Input: part model. Units: mm. Frame: model coordinates. Face numbers are marked on the shaded views. A direction names the side the tool comes from. Give positions to 0.01 mm unless a question says otherwise; leave off trailing zeros. Loops run counter-clockwise (first coordinate to the right, second up) from the corner with the lowest first, then second, coordinate; pieces in that order, holes last. Notation, with made-up numbers: M 37.25,42.25 L 61.25,42.25 A15 cw 61.25,49.25 Z; hole C 18.25,17 d1. An arc over 180 degrees is marked long. One line per item, written item: value. Start each with the question number.
(1) Section B-B on z = 35.5. Output: boundary loops of the cut face in (x, y) (3 decimals), plus the area to 3 significant figures.
(2) Section A-A on y = 25.5. Output: boundary loops of the cut face in (x, z), plus the area to 3 significant figures.
(3) Pull-direction query (Y, two-part tool) for the marked faces 1, 2 and 3; classes: released by +Y, released by -Y, zero draft, split by the parting line, or undercut.
(4) Access query for the marked faces 4, 5 and 6. Directions: +Z, -Z, +X, -X, +Y, -Y. A direction counts if a zero-diameter tool reaches every point of the face in a straight line with its end or side. Return the directions, or none.
(5) Section C-C on x = 16. Output: boundary loops of the cut face in (y, z), plus the area to 3 significant figures.
(6) Pin query (flat end, axial travel): P1, Ø3, axis at y = 7, z = 53.5, coming from the -X side; P2, Ø7.5, axis at x = -30.988, y = 69.088, coming from the +Z side; P3, Ø5.5, axis at x = -30.99, y = -69.09, coming from the -Z side; P4, Ø1.4, axis at x = -6, z = -46.5, coming from the -Y side. Return the tip coordinate at first contact, or that it passes through.
(7) Ray query, line 1 along Y through (x, z) = (0, 145); line 2 along Y through (x, z) = (0, -23); line 3 along Z through (x, y) = (31, -51). Return the intervals inside material, ascending. Write a range as from..to.
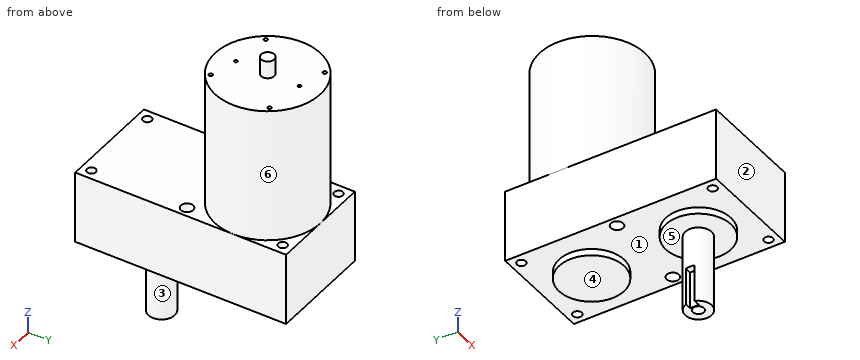
```python
from build123d import *

# Parameters (mm, degrees)
SKETCH1_W                 = 76.2
SKETCH1_H                 = 152.4
SKETCH1_R                 = 4.445
SKETCH1_R_2               = 3.175
SKETCH1_R_3               = 23.495
SKETCH1_R_4               = 9.525
SKETCH1_R_5               = 3.96875
BOSS_EXTRUDE1_DEPTH       = 52.324
SKETCH1_3_R               = 23.495
SKETCH1_3_R_2             = 9.525
BOSS_EXTRUDE2_DEPTH       = 4.826
SKETCH1_5_R               = 9.525
SKETCH1_5_R_2             = 3.96875
BOSS_EXTRUDE3_DEPTH       = 60.198
CUT_EXTRUDE1_START        = -26.924
CUT_EXTRUDE1_DEPTH        = 26.924
SKETCH4_R                 = 38.1
BOSS_EXTRUDE4_DEPTH       = 97.536
SKETCH5_R                 = 4.7625
BOSS_EXTRUDE5_DEPTH       = 12.7
F_4_40_TAPPED_HOLE1_D     = 2.2606
F_4_40_TAPPED_HOLE1_DEPTH = 7.6
F_4_40_TAPPED_HOLE1_TIP   = 0.679152758
F_6_32_TAPPED_HOLE1_D     = 2.7051
F_6_32_TAPPED_HOLE1_DEPTH = 9.39
F_6_32_TAPPED_HOLE1_TIP   = 0.81269403


with BuildPart() as part:
    # Sketch1 → Boss-Extrude1 (new body)
    # profile 1 of 5: a face of its own
    with BuildSketch(Plane.XY):
        Rectangle(SKETCH1_W, SKETCH1_H)
        with Locations((30.988, 0)):
            Circle(SKETCH1_R, mode=Mode.SUBTRACT)
        with Locations((-30.988, 69.088)):
            Circle(SKETCH1_R_2, mode=Mode.SUBTRACT)
        with Locations((-30.994242086, -69.088)):
            Circle(SKETCH1_R_2, mode=Mode.SUBTRACT)
        with Locations((0, 38.608)):
            Circle(SKETCH1_R_3, mode=Mode.SUBTRACT)
        with Locations((0, -38.608)):
            Circle(SKETCH1_R_3, mode=Mode.SUBTRACT)
        with Locations((-30.988, 0)):
            Circle(SKETCH1_R, mode=Mode.SUBTRACT)
        with Locations((30.994242086, -69.088)):
            Circle(SKETCH1_R_2, mode=Mode.SUBTRACT)
        with Locations((30.988, 69.088)):
            Circle(SKETCH1_R_2, mode=Mode.SUBTRACT)
    # profile 2 of 5: a face of its own
    with BuildSketch(Plane.XY):
        with Locations((0, 38.608)):
            Circle(SKETCH1_R_3)
    # profile 3 of 5: a face of its own
    with BuildSketch(Plane.XY):
        with Locations((0, -38.608)):
            Circle(SKETCH1_R_3)
        with Locations((0, -38.608)):
            Circle(SKETCH1_R_4, mode=Mode.SUBTRACT)
    # profile 4 of 5: a face of its own
    with BuildSketch(Plane.XY):
        with Locations((0, -38.608)):
            Circle(SKETCH1_R_4)
        with Locations((0, -38.608)):
            Circle(SKETCH1_R_5, mode=Mode.SUBTRACT)
    # profile 5 of 5: a face of its own
    with BuildSketch(Plane.XY):
        with Locations((0, -38.608)):
            Circle(SKETCH1_R_5)
    extrude(amount=BOSS_EXTRUDE1_DEPTH)

    # Sketch1_3 → Boss-Extrude2 (add)
    # profile 1 of 2: a face of its own
    with BuildSketch(Plane.XY):
        with Locations((0, 38.608)):
            Circle(SKETCH1_3_R)
    # profile 2 of 2: a face of its own
    with BuildSketch(Plane.XY):
        with Locations((0, -38.608)):
            Circle(SKETCH1_3_R)
        with Locations((0, -38.608)):
            Circle(SKETCH1_3_R_2, mode=Mode.SUBTRACT)
    extrude(amount=-BOSS_EXTRUDE2_DEPTH)

    # Sketch1_5 → Boss-Extrude3 (add)
    with BuildSketch(Plane.XY):
        with Locations((0, -38.608)):
            Circle(SKETCH1_5_R)
        with Locations((0, -38.608)):
            Circle(SKETCH1_5_R_2, mode=Mode.SUBTRACT)
    extrude(amount=-BOSS_EXTRUDE3_DEPTH)

    # Sketch2 → Cut-Extrude1 (cut)
    with BuildSketch(Plane(origin=(0, 0, -60.198), x_dir=(-1, 0, 0), z_dir=(0, 0, -1)).offset(CUT_EXTRUDE1_START)):
        with BuildLine():
            Line((8.980256121, -35.433), (4.427938354, -35.433))
            Line((4.427938354, -35.433), (4.427938354, -41.783))
            Line((4.427938354, -41.783), (8.980256121, -41.783))
            ThreePointArc((8.980256121, -41.783), (9.525, -38.608), (8.980256121, -35.433))
        make_face()
    extrude(amount=CUT_EXTRUDE1_DEPTH, mode=Mode.SUBTRACT)

    # Sketch4 → Boss-Extrude4 (add)
    with BuildSketch(Plane.XY.offset(52.324)):
        with Locations((0, 38.1)):
            Circle(SKETCH4_R)
    extrude(amount=BOSS_EXTRUDE4_DEPTH)

    # Sketch5 → Boss-Extrude5 (add)
    with BuildSketch(Plane.XY.offset(149.86)):
        with Locations((0, 38.1)):
            Circle(SKETCH5_R)
    extrude(amount=BOSS_EXTRUDE5_DEPTH)

    # 4-40 Tapped Hole1
    with Locations(Plane.XY.offset(149.86)):
        with Locations((0, 61.1), (0, 15.1)):
            Hole(F_4_40_TAPPED_HOLE1_D / 2, depth=F_4_40_TAPPED_HOLE1_DEPTH)
            with Locations((0, 0, -(F_4_40_TAPPED_HOLE1_DEPTH + F_4_40_TAPPED_HOLE1_TIP / 2))):  # 118° drill point
                Cone(0, F_4_40_TAPPED_HOLE1_D / 2, F_4_40_TAPPED_HOLE1_TIP, mode=Mode.SUBTRACT)

    # 6-32 Tapped Hole1
    with Locations(Plane.XY.offset(149.86)):
        with Locations((28.296788218, 57.913624417), (19.813624417, 9.803211782), (-28.296788218, 18.286375583), (-19.813624417, 66.396788218)):
            Hole(F_6_32_TAPPED_HOLE1_D / 2, depth=F_6_32_TAPPED_HOLE1_DEPTH)
            with Locations((0, 0, -(F_6_32_TAPPED_HOLE1_DEPTH + F_6_32_TAPPED_HOLE1_TIP / 2))):  # 118° drill point
                Cone(0, F_6_32_TAPPED_HOLE1_D / 2, F_6_32_TAPPED_HOLE1_TIP, mode=Mode.SUBTRACT)


solid = part.part
```
Output values:
1. outline: M -38.1,-76.2 L 38.1,-76.2 L 38.1,76.2 L -38.1,76.2 Z; hole C -30.988,0 d8.89; hole C -30.994,-69.088 d6.35; hole C -30.988,69.088 d6.35; hole C 30.988,0 d8.89; hole C 30.988,69.088 d6.35; hole C 30.994,-69.088 d6.35
1. area: 11,400 mm²
2. outline: M -38.1,0 L -19.5,0 L -19.5,-4.83 L 19.5,-4.83 L 19.5,0 L 38.1,0 L 38.1,52.32 L 35.96,52.32 L 35.96,149.86 L -35.96,149.86 L -35.96,52.32 L -38.1,52.32 Z
2. area: 11,200 mm²
3. face 1: undercut
3. face 2: released by -Y
3. face 3: split by the parting line
4. face 4: -Z, +X, -X, +Y
4. face 5: -Z
4. face 6: +Z
5. outline: M -76.2,0 L -55.81,0 L -55.81,-4.83 L -21.4,-4.83 L -21.4,0 L 21.4,0 L 21.4,-4.83 L 55.81,-4.83 L 55.81,0 L 76.2,0 L 76.2,52.32 L 72.68,52.32 L 72.68,149.86 L 3.52,149.86 L 3.52,52.32 L -76.2,52.32 Z
5. area: 15,100 mm²
6. P1: stops at x = -38.1
6. P2: stops at z = 52.32
6. P3: passes through
6. P4: stops at y = -46.52
7. line 1: y = 0..13.97, 16.23..59.97, 62.23..76.2
7. line 2: y = -48.13..-42.58, -34.64..-29.08
7. line 3: z = 0..52.32
